Check sheet for the drawn part. Datum: minimum x, y, z corner. Units: mm. A direction names the side the tool comes from. Give positions to 0.01 mm unless a question says otherwise; leave off trailing zeros. Loops run counter-clockwise (first coordinate to the right, second up) from the corner with the lowest first, then second, coordinate; pieces in that order, holes last. Notation, with made-up numbers: (88, -10) -> (130, -10) arc R27 ccw to (130, 11) -> close; hole circle Ø8 at (67, -38). An arc over 180 degrees is marked (long way). One line per question, with ' | ' between items.
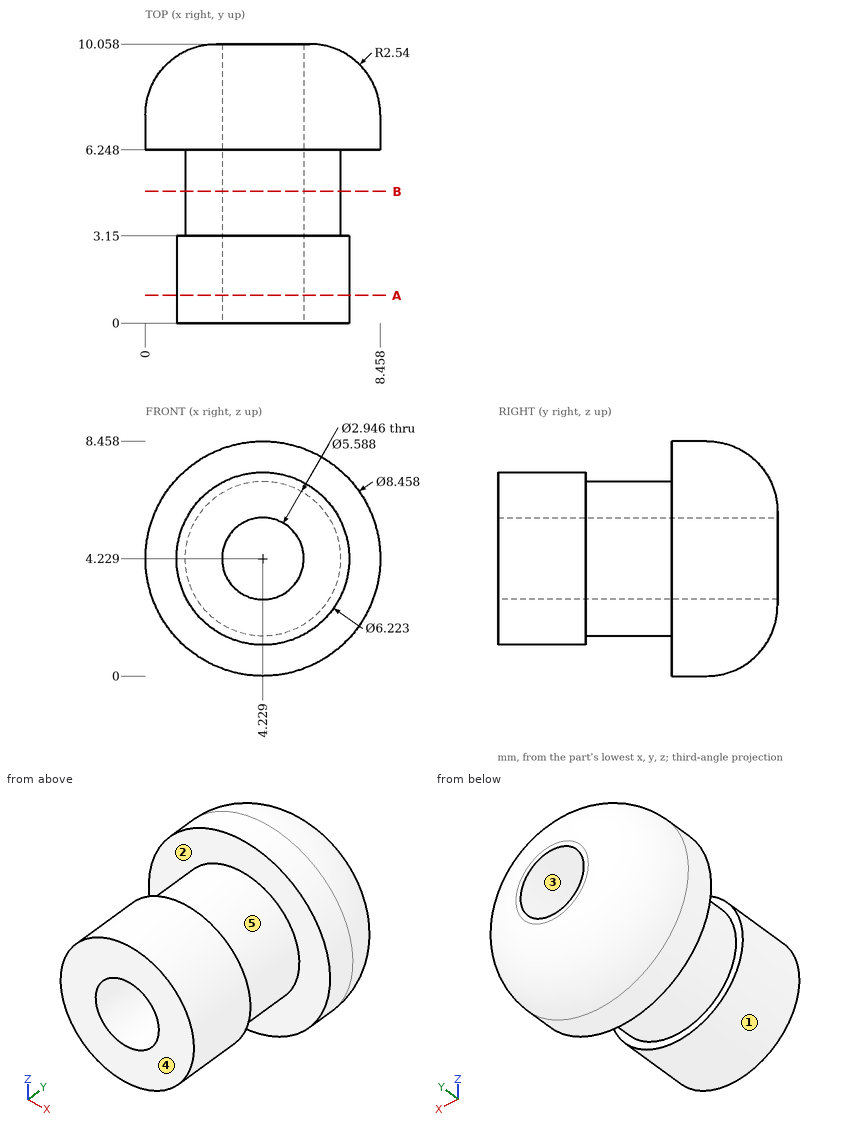
Item 1: Scan lines: probe 1 along Z at (x, y) = (3, 3.25) (1 decimal); probe 2 along X at (y, z) = (4.5, 5.5) (1 decimal); probe 3 along X at (y, z) = (8.75, 5.25) (1 decimal). Record each from-to range of solid material in increasing order.
Result:
probe 1: 1.7 to 3.4, 5 to 6.7 | probe 2: 1.7 to 3.5, 5 to 6.7 | probe 3: 0.5 to 3.2, 5.3 to 8
Item 2: Release check for a two-part mould opening along Z. For the marked faces 1, 2 and 3 record: pulls with the +Z half, pulls with the -Z half, needs draft (parallel to the pull), parting line crosses it, or undercut.
Result:
face 1: parting line crosses it | face 2: needs draft | face 3: undercut
Item 3: Sectioned sample at A-A (y = 1). Record the cut outline in (x, z), plus the area to 3 significant figures.
Result:
outline: circle Ø6.22 at (4.23, 4.23); hole circle Ø2.95 at (4.23, 4.23) | area: 23.6 mm2
Item 4: Depth check by flat-ended pin: pin 1 Ø1 at (y, z) = (9, 4.5) entering from +X; pin 2 Ø2 at (x, z) = (6.5, 1.5) entering from +Y; pin 3 Ø2.5 at (x, z) = (4.23, 4.23) entering from -Y. Enter the tip coordinate at first touch or a pass-through.
Result:
pin 1: x = 8.25 | pin 2: y = 9.91 | pin 3: through
Item 5: Set-up check for the marked faces 4 and 5: record each of +Z, -Z, +X, -X, +Y, -Y from which the full face is reachable in a straight line by a thin tool's end or side.
Result:
face 4: +Z, -Z, +X, -X, -Y | face 5: none
Item 6: Sectioned sample at B-B (y = 4.75). Record the cut outline in (x, z), plus the area to 3 significant figures.
Result:
outline: circle Ø5.59 at (4.23, 4.23); hole circle Ø2.95 at (4.23, 4.23) | area: 17.7 mm2
